For this review, take the finished solid that the model builds, in its own axes (mm). A direction names the side the tool comes from. Give positions to 0.01 mm unless a question says otherwise; leave off trailing zeros. Order: outer loops, then holes, each group sorted by start corner. A loop starts at its lowest first (then second) coordinate and runs counter-clockwise, first axis right, second up. Notation, with made-up numbers: (52, -10.5) - (72, -10.5) arc R32 ccw to (72, 16.5) - close; hole circle Ø5 at (-1.75, 41). An arc over 180 degrees is marked (long way). One line per item, written item: value.
```python
from build123d import *

# Parameters (mm, degrees)
SKETCH2_W           = 60
SKETCH2_H           = 60
BOSS_EXTRUDE1_DEPTH = 2.5
SKETCH3_W           = 2.5
SKETCH3_H           = 12
BOSS_EXTRUDE3_DEPTH = 7
SKETCH6_R           = 1.25
CUT_EXTRUDE1_DEPTH  = 11
CUT_EXTRUDE2_REACH  = 4.5
SKETCH7_R           = 1.5


with BuildPart() as part:
    # Sketch2 → Boss-Extrude1 (new body)
    with BuildSketch(Plane(origin=(0, 0, 0), x_dir=(1, 0, 0), z_dir=(0, 1, 0))):
        Rectangle(SKETCH2_W, SKETCH2_H)
    extrude(amount=BOSS_EXTRUDE1_DEPTH)

    # Sketch3 → Boss-Extrude3 (add)
    with BuildSketch(Plane(origin=(0, 2.5, 0), x_dir=(1, 0, 0), z_dir=(0, 1, 0))):
        with Locations((-4.25, 0)):
            Rectangle(SKETCH3_W, SKETCH3_H)
        with Locations((4.25, 0)):
            Rectangle(SKETCH3_W, SKETCH3_H)
    extrude(amount=BOSS_EXTRUDE3_DEPTH)

    # Sketch6 → Cut-Extrude1 (cut)
    with BuildSketch(Plane.ZY.offset(5.5)):
        with Locations((-3, 6)):
            Circle(SKETCH6_R)
        with Locations((3, 6)):
            Circle(SKETCH6_R)
    extrude(amount=-CUT_EXTRUDE1_DEPTH, mode=Mode.SUBTRACT)

    # Sketch7 → Cut-Extrude2 (cut, up to next)
    with BuildSketch(Plane(origin=(0, 2.5, 0), x_dir=(1, 0, 0), z_dir=(0, 1, 0)), mode=Mode.PRIVATE) as cut_extrude2_sk1:
        with Locations((24, -24)):
            Circle(SKETCH7_R)
    cut_extrude2_tool1 = extrude(cut_extrude2_sk1.sketch, amount=-CUT_EXTRUDE2_REACH, mode=Mode.PRIVATE) & part.part
    add(cut_extrude2_tool1.solids().sort_by_distance((24, 2.5, 24))[0], mode=Mode.SUBTRACT)
    # Sketch7 → Cut-Extrude2 (cut, up to next)
    with BuildSketch(Plane(origin=(0, 2.5, 0), x_dir=(1, 0, 0), z_dir=(0, 1, 0)), mode=Mode.PRIVATE) as cut_extrude2_sk2:
        with Locations((-24, -24)):
            Circle(SKETCH7_R)
    cut_extrude2_tool2 = extrude(cut_extrude2_sk2.sketch, amount=-CUT_EXTRUDE2_REACH, mode=Mode.PRIVATE) & part.part
    add(cut_extrude2_tool2.solids().sort_by_distance((-24, 2.5, 24))[0], mode=Mode.SUBTRACT)
    # Sketch7 → Cut-Extrude2 (cut, up to next)
    with BuildSketch(Plane(origin=(0, 2.5, 0), x_dir=(1, 0, 0), z_dir=(0, 1, 0)), mode=Mode.PRIVATE) as cut_extrude2_sk3:
        with Locations((-24, 24)):
            Circle(SKETCH7_R)
    cut_extrude2_tool3 = extrude(cut_extrude2_sk3.sketch, amount=-CUT_EXTRUDE2_REACH, mode=Mode.PRIVATE) & part.part
    add(cut_extrude2_tool3.solids().sort_by_distance((-24, 2.5, -24))[0], mode=Mode.SUBTRACT)
    # Sketch7 → Cut-Extrude2 (cut, up to next)
    with BuildSketch(Plane(origin=(0, 2.5, 0), x_dir=(1, 0, 0), z_dir=(0, 1, 0)), mode=Mode.PRIVATE) as cut_extrude2_sk4:
        with Locations((24, 24)):
            Circle(SKETCH7_R)
    cut_extrude2_tool4 = extrude(cut_extrude2_sk4.sketch, amount=-CUT_EXTRUDE2_REACH, mode=Mode.PRIVATE) & part.part
    add(cut_extrude2_tool4.solids().sort_by_distance((24, 2.5, -24))[0], mode=Mode.SUBTRACT)
    # Sketch7 → Cut-Extrude2 (cut, up to next)
    with BuildSketch(Plane(origin=(0, 2.5, 0), x_dir=(1, 0, 0), z_dir=(0, 1, 0)), mode=Mode.PRIVATE) as cut_extrude2_sk5:
        with Locations((24, 0)):
            Circle(SKETCH7_R)
    cut_extrude2_tool5 = extrude(cut_extrude2_sk5.sketch, amount=-CUT_EXTRUDE2_REACH, mode=Mode.PRIVATE) & part.part
    add(cut_extrude2_tool5.solids().sort_by_distance((24, 2.5, 0))[0], mode=Mode.SUBTRACT)
    # Sketch7 → Cut-Extrude2 (cut, up to next)
    with BuildSketch(Plane(origin=(0, 2.5, 0), x_dir=(1, 0, 0), z_dir=(0, 1, 0)), mode=Mode.PRIVATE) as cut_extrude2_sk6:
        with Locations((-24, 0)):
            Circle(SKETCH7_R)
    cut_extrude2_tool6 = extrude(cut_extrude2_sk6.sketch, amount=-CUT_EXTRUDE2_REACH, mode=Mode.PRIVATE) & part.part
    add(cut_extrude2_tool6.solids().sort_by_distance((-24, 2.5, 0))[0], mode=Mode.SUBTRACT)
    # Sketch7 → Cut-Extrude2 (cut, up to next)
    with BuildSketch(Plane(origin=(0, 2.5, 0), x_dir=(1, 0, 0), z_dir=(0, 1, 0)), mode=Mode.PRIVATE) as cut_extrude2_sk7:
        with Locations((0, -24)):
            Circle(SKETCH7_R)
    cut_extrude2_tool7 = extrude(cut_extrude2_sk7.sketch, amount=-CUT_EXTRUDE2_REACH, mode=Mode.PRIVATE) & part.part
    add(cut_extrude2_tool7.solids().sort_by_distance((0, 2.5, 24))[0], mode=Mode.SUBTRACT)
    # Sketch7 → Cut-Extrude2 (cut, up to next)
    with BuildSketch(Plane(origin=(0, 2.5, 0), x_dir=(1, 0, 0), z_dir=(0, 1, 0)), mode=Mode.PRIVATE) as cut_extrude2_sk8:
        with Locations((0, 24)):
            Circle(SKETCH7_R)
    cut_extrude2_tool8 = extrude(cut_extrude2_sk8.sketch, amount=-CUT_EXTRUDE2_REACH, mode=Mode.PRIVATE) & part.part
    add(cut_extrude2_tool8.solids().sort_by_distance((0, 2.5, -24))[0], mode=Mode.SUBTRACT)


solid = part.part
```
(1) Machinability: for faces 4 (the face through (-4, 6, 6)), 5 (the face through (-3, 6, 0)), 6 (the face through (-5.5, 6, 0)), 7 (the face through (0, 1, 30)), which of the approach directions +Z, -Z, +X, -X, +Y, -Y give a long, thin tool a straight path to every point of the face, cutting with its end or side? Answer none if there is none.
Answers below:
face 4: +Z, +X, -X, +Y
face 5: +Z, -Z, +Y
face 6: +Z, -Z, -X, +Y
face 7: +Z, +X, -X, +Y, -Y
(2) Take a section at B-B (x = 24). Write out the cut boundary in (y, z), then the cut area to 4 significant figures.
Answers below:
outline: (0, -30) - (2.5, -30) - (2.5, -25.5) - (0, -25.5) - close; (0, -22.5) - (2.5, -22.5) - (2.5, -1.5) - (0, -1.5) - close; (0, 1.5) - (2.5, 1.5) - (2.5, 22.5) - (0, 22.5) - close; (0, 25.5) - (2.5, 25.5) - (2.5, 30) - (0, 30) - close
area: 127.5 mm^2
(3) Take a section at C-C (z = 0). Write out the cut boundary in (x, y).
Answers below:
outline: (-30, 0) - (-25.5, 0) - (-25.5, 2.5) - (-30, 2.5) - close; (-22.5, 0) - (22.5, 0) - (22.5, 2.5) - (5.5, 2.5) - (5.5, 9.5) - (3, 9.5) - (3, 2.5) - (-3, 2.5) - (-3, 9.5) - (-5.5, 9.5) - (-5.5, 2.5) - (-22.5, 2.5) - close; (25.5, 0) - (30, 0) - (30, 2.5) - (25.5, 2.5) - close
(4) Draft analysis for pull direction Z (two halves, no side actions). For faces 1 (the face through (22.89, 1.27, 22.99)), 2 (the face through (4, 6, 6)), 3 (the face through (0, 1, -30)), state which applies: pulls with the +Z half, pulls with the -Z half, needs draft (parallel to the pull), parting line crosses it, or undercut.
Answers below:
face 1: undercut
face 2: pulls with the +Z half
face 3: pulls with the -Z half
(5) Take a section at A-A (y = 6). Write out the cut boundary in (x, z), then the cut area to 3 significant figures.
Answers below:
outline: (-5.5, -6) - (-3, -6) - (-3, -4.25) - (-5.5, -4.25) - close; (-5.5, -1.75) - (-3, -1.75) - (-3, 1.75) - (-5.5, 1.75) - close; (-5.5, 4.25) - (-3, 4.25) - (-3, 6) - (-5.5, 6) - close; (3, -6) - (5.5, -6) - (5.5, -4.25) - (3, -4.25) - close; (3, -1.75) - (5.5, -1.75) - (5.5, 1.75) - (3, 1.75) - close; (3, 4.25) - (5.5, 4.25) - (5.5, 6) - (3, 6) - close
area: 35.0 mm^2
(6) Wall thickness on line 1 (Z direction, x = -24, y = 2.05); line 2 (Z direction, x = 0, y = 1.8): over which ranges is each line inside the solid? List them lowest first. Write a range as from..to.
Answers below:
line 1: z = -30..-25.5, -22.5..-1.5, 1.5..22.5, 25.5..30
line 2: z = -30..-25.5, -22.5..22.5, 25.5..30
(7) Take a section at D-D (y = 1.75). Give the number of separate pieces and of enclosed holes in the cut face, then the cut area to 3 significant figures.
Answers below:
separate pieces: 1
enclosed holes: 8
area: 3,540 mm^2
(8) For P1, Ø2, axis at y = 6, z = 3, coming from the +X side; P2, Ø3.5, axis at y = 4.5, z = 2, coming from the +X side; P3, Ø8, axis at x = 16.5, z = 5, coming from the +Y side; P4, Ø1, axis at x = 4, y = 7.5, coming from the +Z side, all flat-tipped, find the tip position at first contact; note any pin that passes through.
Answers below:
P1: passes through
P2: stops at x = 5.5
P3: stops at y = 2.5
P4: stops at z = 6
